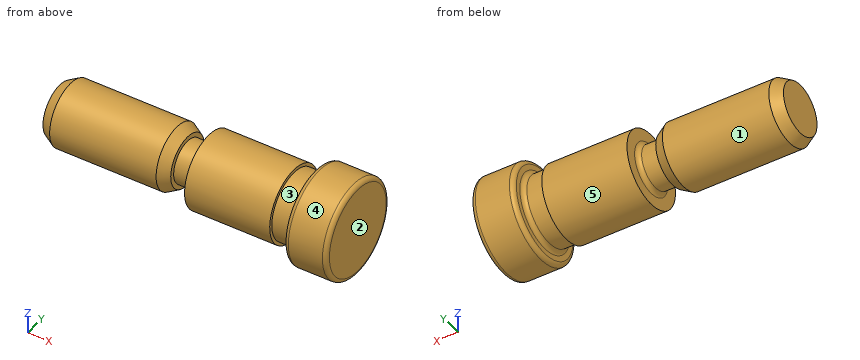
```python
from build123d import *

# Parameters (mm, degrees)
F2_SIZE2 = 2.8867513459
F2_SIZE  = 5
F3_R     = 2


with BuildPart() as f1:
    # F0 (on Front) → F1 (revolve)
    with BuildSketch(Plane.XZ):
        Polygon((-140, 0), (0, 0), (0, 22.5), (-20, 22.5), (-20, 16), (-30, 16), (-30, 17.5), (-70, 17.5), (-70, 10), (-80, 10), (-80, 15), (-140, 15), align=None)
    revolve(axis=Axis((-70, 0, 0), (1, 0, 0)))

    # F2
    f2_edges = [f1.edges().sort_by_distance(p)[0] for p in [
        (-140, 0, -15),
        (-80, 0, -15),
    ]]
    f2_side = f1.faces().sort_by_distance((-110, 0, -15))[0]
    chamfer(f2_edges, length=F2_SIZE, length2=F2_SIZE2, reference=f2_side)

    # F3
    f3_edges = [f1.edges().sort_by_distance(p)[0] for p in [
        (-70, 0, -10),
        (-20, 0, -22.5),
        (0, 0, -22.5),
        (-20, 0, -16),
    ]]
    fillet(f3_edges, radius=F3_R)


solid = f1.part
```
The model under review builds one solid part; all positions refer to its coordinate system, in mm. Face numbers are marked on the shaded views. A direction names the side the tool comes from. Round coordinates to 2 decimals unless told otherwise and drop trailing zeros. Loops run counter-clockwise (first coordinate to the right, second up) from the corner with the lowest first, then second, coordinate; pieces in that order, holes last. Notation, with made-up numbers: M 50.5,64 L 81.5,64 A17 ccw 81.5,89 Z; hole C 79.5,-27.5 d9. An arc over 180 degrees is marked long. Write item = value, one per line.
Item 1: Take a section at C-C on x = -106.5. Write out the cut boundary in (y, z).
Return value:
outline = C 0,0 d30
Item 2: Insertion check: P1, Ø6, axis at x = -62.5, z = -13, coming from the +Y side; P2, Ø1.5, axis at x = -58, y = -4, coming from the -Z side; P3, Ø4, axis at x = -51, y = 15, coming from the +Z side. Each pin has a flat end and moves straight along its axis. Give the tip position at first contact, or say it passes through.
Return value:
P1 = 14.36
P2 = -17.2
P3 = 11.72
Item 3: Machinability: for the marked faces 4 and 5, which of the approach directions +Z, -Z, +X, -X, +Y, -Y give a long, thin tool a straight path to every point of the face, cutting with its end or side? Answer none if there is none.
Return value:
face_4 = +X, -X
face_5 = -X
Item 4: For line 1 (X direction, y = 10, z = 6); line 2 (X direction, y = 11.5, z = -14.5); line 3 (X direction, y = -5, z = -15), list the stretches that pass through material, from the lowest coordinate up. Write a range as [from, to].
Return value:
line_1 = [-140, -80], [-70.03, 0]
line_2 = [-20, 0]
line_3 = [-70, 0]
Item 5: The part is to be moulded in two halves that separate along X. For the marked faces 1, 2 and 3, say which applies: released by +X, released by -X, zero draft, split by the parting line, or undercut.
Return value:
face_1 = zero draft
face_2 = released by +X
face_3 = undercut
Item 6: Take a section at D-D on x = -56.5. Write out the cut boundary in (y, z).
Return value:
outline = C 0,0 d35
